The listing builds one solid part. Answer for the finished solid, in the listing's coordinates (mm). Face numbers are marked on the shaded views. A direction names the side the tool comes from. Round coordinates to 2 decimals unless told otherwise and drop trailing zeros. Return JSON: item names as keys, results as strings. Group by question number.
(1) The part is cut by section A-A (x = 0). Count the separate pieces of the cut face and the enclosed holes in it, plus the area to 3 significant figures.
(2) Consider line 1 (Y direction, x = 34.5, z = 1.75); line 2 (Y direction, x = 48, z = 1.75); line 3 (Y direction, x = 16, z = 5.25). Determine where each line is inside the solid, lowest interval first. Write a range as [from, to].
(3) Each of these flat-tipped pins is pushed along its axis until it touches: pin 1 (1.5 mm diameter, centred on x = 50.5, z = 6.5, fed in from +Y); pin 2 (19 mm diameter, centred on x = -17.32, y = 10, fed in from -Z); pin 3 (17 mm diameter, centred on x = 0, y = 0, fed in from +Z); pin 4 (6 mm diameter, centred on y = 19, z = 4.5, fed in from -X). Where does it stop, or does it pass through?
(4) Which of the six approach directions +Z, -Z, +X, -X, +Y, -Y give full straight-line access (tool end or side, diameter ignored) to the marked faces 4, 5, 6 and 7?
(5) Determine the mould class of the marked faces 1, 2 and 3 for opening direction X: +X half, -X half, draft (parallel to the pull), parting line (faces both ways), or undercut.
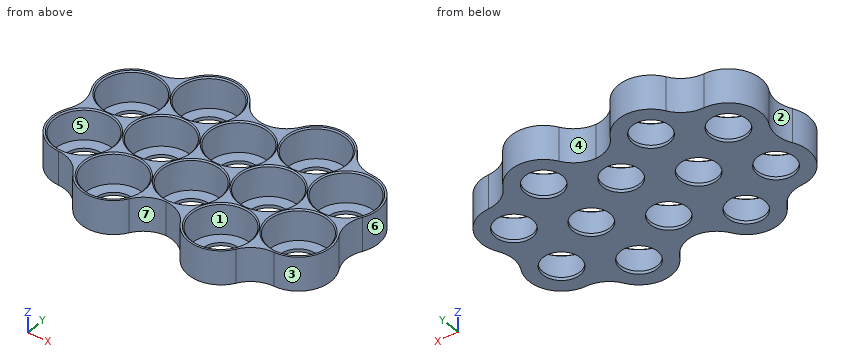
from build123d import *

# Parameters (mm, degrees)
F0_R        = 9.5
F1_DEPTH    = 11
F0_R_2      = 6
F2_DEPTH    = 1
F3_T1_DEPTH = 11
F4_SIZE     = 0.4


# Not quite as in the source:
# - a fillet or chamfer that OpenCascade refuses, or shapes differently, is made with other operations: its cross-section is extruded or revolved along the edge and cut away or added


with BuildPart() as f1:
    # F0 (on Top) → F1 (new body)
    with BuildSketch(Plane.XY):
        with BuildLine():
            ThreePointArc((10.2610350972, 17.7726341266), (0, 30.5), (-10.2610350972, 17.7726341266))
            ThreePointArc((-10.2610350972, 17.7726341266), (-26.4137748154, 15.25), (-20.5220701944, 0))
            ThreePointArc((-20.5220701944, 0), (-26.4137748154, -15.25), (-10.2610350972, -17.7726341266))
            ThreePointArc((-10.2610350972, -17.7726341266), (0, -30.5), (10.2610350972, -17.7726341266))
            ThreePointArc((10.2610350972, -17.7726341266), (17.3205080757, -20.5), (24.3799810542, -17.7726341266))
            ThreePointArc((24.3799810542, -17.7726341266), (34.6410161514, -30.5), (44.9020512486, -17.7726341266))
            ThreePointArc((44.9020512486, -17.7726341266), (61.0547909668, -15.25), (55.1630863458, 0))
            ThreePointArc((55.1630863458, 0), (61.0547909668, 15.25), (44.9020512486, 17.7726341266))
            ThreePointArc((44.9020512486, 17.7726341266), (34.6410161514, 30.5), (24.3799810542, 17.7726341266))
            ThreePointArc((24.3799810542, 17.7726341266), (17.3205080757, 20.5), (10.2610350972, 17.7726341266))
        make_face()
        with Locations((0, -20)):
            Circle(F0_R, mode=Mode.SUBTRACT)
        with Locations((-17.3205080757, -10)):
            Circle(F0_R, mode=Mode.SUBTRACT)
        with Locations((34.6410161514, -20)):
            Circle(F0_R, mode=Mode.SUBTRACT)
        with Locations((17.3205080757, -10)):
            Circle(F0_R, mode=Mode.SUBTRACT)
        with Locations((51.9615242271, -10)):
            Circle(F0_R, mode=Mode.SUBTRACT)
        with Locations((-17.3205080757, 10)):
            Circle(F0_R, mode=Mode.SUBTRACT)
        Circle(F0_R, mode=Mode.SUBTRACT)
        with Locations((0, 20)):
            Circle(F0_R, mode=Mode.SUBTRACT)
        with Locations((34.6410161514, 0)):
            Circle(F0_R, mode=Mode.SUBTRACT)
        with Locations((17.3205080757, 10)):
            Circle(F0_R, mode=Mode.SUBTRACT)
        with Locations((51.9615242271, 10)):
            Circle(F0_R, mode=Mode.SUBTRACT)
        with Locations((34.6410161514, 20)):
            Circle(F0_R, mode=Mode.SUBTRACT)
    extrude(amount=F1_DEPTH)

    # F0 (on Top) → F2 (join)
    with BuildSketch(Plane.XY):
        with Locations((0, 20)):
            Circle(F0_R)
        with Locations((0, 20)):
            Circle(F0_R_2, mode=Mode.SUBTRACT)
        with Locations((-17.3205080757, 10)):
            Circle(F0_R)
        with Locations((-17.3205080757, 10)):
            Circle(F0_R_2, mode=Mode.SUBTRACT)
        with Locations((-17.3205080757, -10)):
            Circle(F0_R)
        with Locations((-17.3205080757, -10)):
            Circle(F0_R_2, mode=Mode.SUBTRACT)
        Circle(F0_R)
        Circle(F0_R_2, mode=Mode.SUBTRACT)
        with Locations((0, -20)):
            Circle(F0_R)
        with Locations((0, -20)):
            Circle(F0_R_2, mode=Mode.SUBTRACT)
        with Locations((17.3205080757, -10)):
            Circle(F0_R)
        with Locations((17.3205080757, -10)):
            Circle(F0_R_2, mode=Mode.SUBTRACT)
        with Locations((17.3205080757, 10)):
            Circle(F0_R)
        with Locations((17.3205080757, 10)):
            Circle(F0_R_2, mode=Mode.SUBTRACT)
        with Locations((34.6410161514, 20)):
            Circle(F0_R)
        with Locations((34.6410161514, 20)):
            Circle(F0_R_2, mode=Mode.SUBTRACT)
        with Locations((34.6410161514, 0)):
            Circle(F0_R)
        with Locations((34.6410161514, 0)):
            Circle(F0_R_2, mode=Mode.SUBTRACT)
        with Locations((34.6410161514, -20)):
            Circle(F0_R)
        with Locations((34.6410161514, -20)):
            Circle(F0_R_2, mode=Mode.SUBTRACT)
        with Locations((51.9615242271, -10)):
            Circle(F0_R)
        with Locations((51.9615242271, -10)):
            Circle(F0_R_2, mode=Mode.SUBTRACT)
        with Locations((51.9615242271, 10)):
            Circle(F0_R)
        with Locations((51.9615242271, 10)):
            Circle(F0_R_2, mode=Mode.SUBTRACT)
    extrude(amount=F2_DEPTH)

    # F3: fillet of radius 10 on 10 edges, made by hand

    # F3_s2 → F3_t1 (join)
    with BuildSketch(Plane.XY):
        with BuildLine():
            ThreePointArc((25.6222746499, 25.3770160619), (22.0329970294, 21.837729702), (17.1732463203, 20.4989672814))
            ThreePointArc((17.1732463203, 20.4989672814), (21.0357320415, 19.8207489981), (24.3799810542, 17.7726341266))
            ThreePointArc((24.3799810542, 17.7726341266), (24.2783860519, 21.692896164), (25.6222746499, 25.3770160619))
        make_face()
        with BuildLine():
            ThreePointArc((17.4677698311, 20.4989672814), (12.6080191219, 21.837729702), (9.0187415015, 25.3770160619))
            ThreePointArc((9.0187415015, 25.3770160619), (10.3626300995, 21.692896164), (10.2610350972, 17.7726341266))
            ThreePointArc((10.2610350972, 17.7726341266), (13.6052841099, 19.8207489981), (17.4677698311, 20.4989672814))
        make_face()
        with BuildLine():
            ThreePointArc((-9.0187415015, 25.3770160619), (-12.6080191219, 21.837729702), (-17.4677698311, 20.4989672814))
            ThreePointArc((-17.4677698311, 20.4989672814), (-13.6052841099, 19.8207489981), (-10.2610350972, 17.7726341266))
            ThreePointArc((-10.2610350972, 17.7726341266), (-10.3626300995, 21.692896164), (-9.0187415015, 25.3770160619))
        make_face()
        with BuildLine():
            ThreePointArc((-26.4865113326, 4.8780487805), (-25.2160382439, 0), (-26.4865113326, -4.8780487805))
            ThreePointArc((-26.4865113326, -4.8780487805), (-23.9679142094, -1.8721471658), (-20.5220701944, 0))
            ThreePointArc((-20.5220701944, 0), (-23.9679142094, 1.8721471658), (-26.4865113326, 4.8780487805))
        make_face()
        with BuildLine():
            ThreePointArc((-17.4677698311, -20.4989672814), (-12.6080191219, -21.837729702), (-9.0187415015, -25.3770160619))
            ThreePointArc((-9.0187415015, -25.3770160619), (-10.3626300995, -21.692896164), (-10.2610350972, -17.7726341266))
            ThreePointArc((-10.2610350972, -17.7726341266), (-13.6052841099, -19.8207489981), (-17.4677698311, -20.4989672814))
        make_face()
        with BuildLine():
            ThreePointArc((9.0187415015, -25.3770160619), (12.6080191219, -21.837729702), (17.4677698311, -20.4989672814))
            ThreePointArc((17.4677698311, -20.4989672814), (13.6052841099, -19.8207489981), (10.2610350972, -17.7726341266))
            ThreePointArc((10.2610350972, -17.7726341266), (10.3626300995, -21.692896164), (9.0187415015, -25.3770160619))
        make_face()
        with BuildLine():
            ThreePointArc((25.6222746499, -25.3770160619), (22.0329970294, -21.837729702), (17.1732463203, -20.4989672814))
            ThreePointArc((17.1732463203, -20.4989672814), (21.0357320415, -19.8207489981), (24.3799810542, -17.7726341266))
            ThreePointArc((24.3799810542, -17.7726341266), (24.2783860519, -21.692896164), (25.6222746499, -25.3770160619))
        make_face()
        with BuildLine():
            ThreePointArc((52.1087859825, -20.4989672814), (47.2490352733, -21.837729702), (43.6597576529, -25.3770160619))
            ThreePointArc((43.6597576529, -25.3770160619), (45.0036462508, -21.692896164), (44.9020512486, -17.7726341266))
            ThreePointArc((44.9020512486, -17.7726341266), (48.2463002613, -19.8207489981), (52.1087859825, -20.4989672814))
        make_face()
        with BuildLine():
            ThreePointArc((61.1275274839, 4.8780487805), (59.8570543952, 0), (61.1275274839, -4.8780487805))
            ThreePointArc((61.1275274839, -4.8780487805), (58.6089303607, -1.8721471658), (55.1630863458, 0))
            ThreePointArc((55.1630863458, 0), (58.6089303607, 1.8721471658), (61.1275274839, 4.8780487805))
        make_face()
        with BuildLine():
            ThreePointArc((52.1087859825, 20.4989672814), (47.2490352733, 21.837729702), (43.6597576529, 25.3770160619))
            ThreePointArc((43.6597576529, 25.3770160619), (45.0036462508, 21.692896164), (44.9020512486, 17.7726341266))
            ThreePointArc((44.9020512486, 17.7726341266), (48.2463002613, 19.8207489981), (52.1087859825, 20.4989672814))
        make_face()
    extrude(amount=F3_T1_DEPTH)

    # F4
    f4_edges = [f1.edges().sort_by_distance(p)[0] for p in [
        (-26.820508, 10, 11),
        (-9.5, 20, 11),
        (-26.820508, -10, 11),
        (-9.5, 0, 11),
        (-9.5, -20, 11),
        (7.820508, -10, 11),
        (7.820508, 10, 11),
        (25.141016, 20, 11),
        (25.141016, 0, 11),
        (42.461524, 10, 11),
        (42.461524, -10, 11),
        (25.141016, -20, 11),
    ]]
    chamfer(f4_edges, length=F4_SIZE)


solid = f1.part
Answer below:
{
 "1": {"separate pieces": "4", "enclosed holes": "0", "area": "64.5 mm²"},
 "2": {"line 1": "y = [-30.5, -29.5], [-10.5, -9.5], [9.5, 10.5], [29.5, 30.5]", "line 2": "y = [-21.45, -18.63], [-1.37, 1.37], [18.63, 21.45]", "line 3": "y = [-20.63, -19.41], [-0.59, 0.59], [19.41, 20.63]"},
 "3": {"pin 1": "stops at y = 20.82", "pin 2": "stops at z = 0", "pin 3": "stops at z = 1", "pin 4": "stops at x = -25.94"},
 "4": {"face 4": "+Z, -Z, +Y", "face 5": "+Z", "face 6": "+Z, -Z, +X", "face 7": "+Z, -Z, -Y"},
 "5": {"face 1": "undercut", "face 2": "-X half", "face 3": "+X half"}
}
